```python
from build123d import *

# Parameters (mm, degrees)
EXTRUDE_1_DEPTH     = 2
EXTRUDE_2_DEPTH     = 10.5
SKETCH_3_R          = 1.95
EXTRUDE_3_DEPTH     = 4
FILLET_1_R          = 3
SKETCH_4_R          = 1.2
CUT_EXTRUDE_1_DEPTH = 28.201889258
SKETCH_5_R          = 2
CUT_EXTRUDE_2_DEPTH = 2.6


with BuildPart() as part:
    # 스케치1 → 보스-돌출1 (new body)
    with BuildSketch(Plane.XY):
        with BuildLine():
            Line((-8.811473671, -9.461920088), (-10.811473671, -12.926021703))
            Line((-10.811473671, -12.926021703), (-5.788526329, -15.826021703))
            Line((-5.788526329, -15.826021703), (5.788526329, -15.826021703))
            Line((5.788526329, -15.826021703), (10.811473671, -12.926021703))
            Line((10.811473671, -12.926021703), (8.811473671, -9.461920088))
            Line((8.811473671, -9.461920088), (5.137782868, -3.098900966))
            ThreePointArc((5.137782868, -3.098900966), (0, 6), (-5.137782868, -3.098900966))
            Line((-5.137782868, -3.098900966), (-8.811473671, -9.461920088))
        make_face()
    extrude(amount=EXTRUDE_1_DEPTH)

    # 스케치2 → 보스-돌출2 (add)
    with BuildSketch(Plane.XY.offset(2)):
        Polygon((-5.788526329, -15.826021703), (-10.811473671, -12.926021703), (-8.811473671, -9.461920088), (-3.788526329, -12.361920088), align=None)
        Polygon((5.788526329, -15.826021703), (3.788526329, -12.361920088), (8.811473671, -9.461920088), (10.811473671, -12.926021703), align=None)
    extrude(amount=EXTRUDE_2_DEPTH)

    # 스케치3 → 보스-돌출3 (add)
    with BuildSketch(Plane.XY.offset(2)):
        Circle(SKETCH_3_R)
    extrude(amount=EXTRUDE_3_DEPTH)

    # 필렛1
    fillet_1_edges = [part.edges().sort_by_distance(p)[0] for p in [
        (-6.3, -10.911920088, 2),
        (6.3, -10.911920088, 2),
    ]]
    fillet(fillet_1_edges, radius=FILLET_1_R)

    # 스케치4 → 컷-돌출1 (cut, through all)
    with BuildSketch(Plane(origin=(-8.3, -14.376021703, 0), x_dir=(0.866025404, -0.5, 0), z_dir=(-0.5, -0.866025404, 0))):
        with Locations((0, 10)):
            Circle(SKETCH_4_R)
    cut_extrude_1 = extrude(amount=-CUT_EXTRUDE_1_DEPTH, mode=Mode.SUBTRACT)

    # 스케치5 → 컷-돌출2 (cut)
    with BuildSketch(Plane(origin=(-8.3, -14.376021703, 0), x_dir=(0.866025404, -0.5, 0), z_dir=(-0.5, -0.866025404, 0))):
        with Locations((0, 10)):
            Circle(SKETCH_5_R)
    cut_extrude_2 = extrude(amount=-CUT_EXTRUDE_2_DEPTH, mode=Mode.SUBTRACT)

    # 대칭 복사1: 컷-돌출1, 컷-돌출2 across plane
    add(cut_extrude_1.mirror(Plane(origin=(0, 0, 0), x_dir=(0, 0, 1), z_dir=(1, 0, 0))), mode=Mode.SUBTRACT)
    add(cut_extrude_2.mirror(Plane(origin=(0, 0, 0), x_dir=(0, 0, 1), z_dir=(1, 0, 0))), mode=Mode.SUBTRACT)


solid = part.part
```
Could you check a few things on this model? Use its own coordinates, in mm. A direction names the side the tool comes from. Coordinates: 2 decimals unless noted, no trailing zeros. Write each loop counter-clockwise with the first axis right and the second up, starting at its lowest first coordinate (ties: lowest second). Pieces come first, ordered by that corner, then holes. Notation, with made-up numbers: M 59,33 L 90,33 A7 ccw 90,40 Z; hole C -21,49.25 d3. An arc over 180 degrees is marked long. Answer as CSV lines item,"result". Start each with the question number.
1) Please list where these lines run through material, in increasing order: line 1 (Z direction, x = -3.25, y = -6); line 2 (X direction, y = -12.75, z = 3.5); line 3 (X direction, y = -12.25, z = 11). Write a range as from..to.
2) We'd pull the mould along X, two halves only. Please class faces 6 (the cylindrical face through (-1.437, 1.318, 3.972)), 7 (the flat face through (-4.79, -14.1, 7.18)), 8 (the flat face through (-6.89, -10.57, 8.7)), 9 (the flat face through (0, 0, 6)): +X half, -X half, draft (parallel to the pull), parting line (faces both ways), or undercut.
3) For faces 1 (the flat face through (7, -13, 12.5)), 2 (the flat face through (4.84, -14.18, 7.18)), 3 (the flat face through (0, -5, 2)), 4 (the flat face through (6.82, -10.61, 8.7)), 5 (the flat face through (-6.64, -12.33, 8.69)), which set-ups out of +Z, -Z, +X, -X, +Y, -Y let a thin tool reach every point of the face, with its end or its side?
4) I want a section at D-D, the plane z = 2.75. Please give me the cut outline in (x, y), and give its area (3 significant figures).
5) I want a section at B-B, the plane z = 7. Please give me the cut outline in (x, y), and give its area (3 significant figures).
6) I want a section at C-C, the plane y = 0. Please give me the cut outline in (x, z).
7) I want a section at A-A, the plane x = 0. Please give me the cut outline in (y, z).
8) For P1, Ø4, axis at x = 1.5, z = 6.5, coming from the -Y side; P2, Ø3, axis at y = -4, z = 8, coming from the +X side; P3, Ø4, axis at x = 2.5, z = 7, coming from the +Y side; P4, Ø4.5, axis at x = 2.5, y = -2, coming from the +Z side, each with a flat end and sliding along its axis, tell me the tip position at first contact or that it passes through.
Data:
1,line 1,"z = 0..2"
1,line 2,"x = -10.71..-4.01, 4.01..10.71"
1,line 3,"x = -10.42..-9.07, -6.31..-3.98, 3.98..6.31, 9.07..10.42"
2,face 6,"parting line"
2,face 7,"undercut"
2,face 8,"undercut"
2,face 9,"draft"
3,face 1,"+Z, +X, -X, +Y, -Y"
3,face 2,"+Z, -Y"
3,face 3,"+Z"
3,face 4,"+Z, +Y"
3,face 5,"none"
4,outline,"M -10.81,-12.93 L -5.79,-15.83 L -3.28,-11.48 L -8.3,-8.58 Z; C 0,0 d3.9; M 3.28,-11.48 L 5.79,-15.83 L 10.81,-12.93 L 8.3,-8.58 Z"
4,area,"70.1 mm^2"
5,outline,"M -10.81,-12.93 L -5.79,-15.83 L -3.79,-12.36 L -8.81,-9.46 Z; M 3.79,-12.36 L 5.79,-15.83 L 10.81,-12.93 L 8.81,-9.46 Z"
5,area,"46.4 mm^2"
6,outline,"M -6,0 L 6,0 L 6,2 L 1.95,2 L 1.95,6 L -1.95,6 L -1.95,2 L -6,2 Z"
7,outline,"M -15.83,0 L 6,0 L 6,2 L 1.95,2 L 1.95,6 L -1.95,6 L -1.95,2 L -15.83,2 Z"
8,P1,"stops at y = -1.95"
8,P2,"passes through"
8,P3,"stops at y = 1.79"
8,P4,"stops at z = 6"
